Check sheet for the modelled part. Datum: model origin and axes. Units: mm. A direction names the side the tool comes from. Round coordinates to 2 decimals unless told otherwise and drop trailing zeros. Order: outer loops, then holes, each group sorted by start corner. A loop starts at its lowest first (then second) coordinate and runs counter-clockwise, first axis right, second up.
Q1. Cross-section at D-D on x = 20.5. Record the cut outline in (y, z), then the cut area to 3 significant figures.
Q2. Scan lines: probe 1 along Z at (x, y) = (20, 2); probe 2 along Y at (x, z) = (100, -4); probe 3 along Z at (x, y) = (30.5, 37.5). Record each from-to range of solid material in increasing order.
Q3. Cross-section at A-A on x = 130. Record the cut outline in (y, z), then the cut area to 3 significant figures.
Q4. Depth check by flat-ended pin: P1, Ø8, axis at x = 17, z = -23.5, coming from the +Y side; P2, Ø16, axis at x = 50, y = 18, coming from the -Z side. Enter the tip coordinate at first touch or a pass-through.
Q5. Cross-section at B-B on y = 18. Record the cut outline in (x, z), then the cut area to 3 significant figures.
Q6. Set-up check for faces 1 (the flat face through (74, 28, -5)), 2 (the cylindrical face through (18.92, 13.12, -2.46)): record each of +Z, -Z, +X, -X, +Y, -Y from which the full face is reachable in a straight line by a thin tool's end or side.
Q7. Mould release check, pull along Z, two halves, no side actions. Record for faces 3 (the cylindrical face through (104.77, 2.46, -35.5)), 4 (the flat face through (74, 25, 0)), 5 (the cylindrical face through (132.307, 13.564, -2.465)): +Z half, -Z half, draft (parallel to the pull), parting line (faces both ways), or undercut.
Q8. Cross-section at C-C on z = -37. Record the cut outline in (x, y), then the cut area to 3 significant figures.
from build123d import *

# Parameters (mm, degrees)
EXTRUDE_1_DEPTH     = 150
SKETCH_2_R          = 5
CUT_EXTRUDE_1_DEPTH = 51
SKETCH_3_R          = 5
CUT_EXTRUDE_3_DEPTH = 51


with BuildPart() as part:
    # Эскиз1 → Вытянуть-Тонкостенный1 (new body)
    with BuildSketch(Plane(origin=(0, 0, 0), x_dir=(0, 0, -1), z_dir=(1, 0, 0))):
        Polygon((50, 0), (0, 0), (0, 50), (5, 50), (5, 5), (50, 5), align=None)
    extrude(amount=EXTRUDE_1_DEPTH)

    # Эскиз2 → Вырез-Вытянуть1 (cut, through all)
    with BuildSketch(Plane.XZ):
        with Locations((130, -37)):
            Circle(SKETCH_2_R)
        with Locations((100, -37)):
            Circle(SKETCH_2_R)
        with Locations((50, -37)):
            Circle(SKETCH_2_R)
        with Locations((20, -37)):
            Circle(SKETCH_2_R)
    extrude(amount=-CUT_EXTRUDE_1_DEPTH, mode=Mode.SUBTRACT)

    # Эскиз3 → Вырез-Вытянуть3 (cut, through all)
    with BuildSketch(Plane.XY):
        with Locations((130, 18)):
            Circle(SKETCH_3_R)
        with Locations((100, 18)):
            Circle(SKETCH_3_R)
        with Locations((50, 18)):
            Circle(SKETCH_3_R)
        with Locations((20, 18)):
            Circle(SKETCH_3_R)
    extrude(amount=-CUT_EXTRUDE_3_DEPTH, mode=Mode.SUBTRACT)


solid = part.part
Results found:
1. outline: (0, -50) - (5, -50) - (5, -41.97) - (0, -41.97) - close; (0, -32.03) - (5, -32.03) - (5, -5) - (13.03, -5) - (13.03, 0) - (0, 0) - close; (22.97, -5) - (50, -5) - (50, 0) - (22.97, 0) - close
1. area: 376 mm2
2. probe 1: z = -50 to -42, -32 to 0
2. probe 2: y = 0 to 13, 23 to 50
2. probe 3: z = -5 to 0
3. outline: (0, -50) - (5, -50) - (5, -42) - (0, -42) - close; (0, -32) - (5, -32) - (5, -5) - (13, -5) - (13, 0) - (0, 0) - close; (23, -5) - (50, -5) - (50, 0) - (23, 0) - close
3. area: 375 mm2
4. P1: stops at y = 5
4. P2: stops at z = -5
5. outline: (0, -5) - (15, -5) - (15, 0) - (0, 0) - close; (25, -5) - (45, -5) - (45, 0) - (25, 0) - close; (55, -5) - (95, -5) - (95, 0) - (55, 0) - close; (105, -5) - (125, -5) - (125, 0) - (105, 0) - close; (135, -5) - (150, -5) - (150, 0) - (135, 0) - close
5. area: 550 mm2
6. face 1: -Z, +X, -X, +Y
6. face 2: +Z, -Z
7. face 3: undercut
7. face 4: +Z half
7. face 5: draft
8. outline: (0, 0) - (15, 0) - (15, 5) - (0, 5) - close; (25, 0) - (45, 0) - (45, 5) - (25, 5) - close; (55, 0) - (95, 0) - (95, 5) - (55, 5) - close; (105, 0) - (125, 0) - (125, 5) - (105, 5) - close; (135, 0) - (150, 0) - (150, 5) - (135, 5) - close
8. area: 550 mm2
